Input: part model. Units: mm. Frame: model coordinates. Give positions to 0.01 mm unless a question says otherwise; leave off trailing zeros. Loops run counter-clockwise (first coordinate to the right, second up) from the corner with the lowest first, then second, coordinate; pieces in that order, holes last. Notation, with made-up numbers: (33.5, 55.25) - (87.5, 55.25) arc R36 cw to (87.5, 93.25) - close; hole circle Ø5 at (-7.5, 62). An arc over 180 degrees is marked (long way). Answer as a JSON object with one key per item and string values. Group by question number.
(1) Pin query (flat end, axial travel): P1, Ø1.8, axis at x = -85, y = 10, coming from the -Z side; P2, Ø2, axis at x = 22, z = 74.5, coming from the +Y side; P3, Ø2.5, axis at y = 13.5, z = 98, coming from the +X side; P4, Ø5, axis at y = 10.5, z = -56.5, coming from the +X side. Return the tip coordinate at first contact, or that it passes through.
(2) Section query B-B (z = 69.5). Return loops of the section in (x, y).
(3) Material intervals for L1, parallel to Y at x = -17.5, z = 97.9; L2, parallel to X at y = 2.3, z = -30; L3, parallel to Y at x = -96.15, z = -90, sorted ascending.
(4) Section query A-A (x = -65.5). Return loops of the section in (y, z).
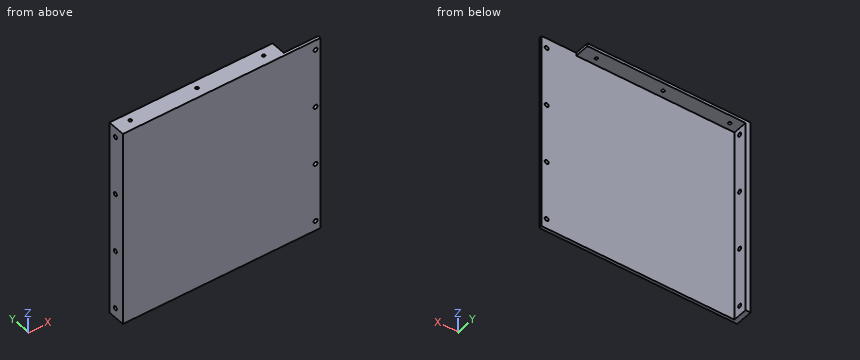
```python
from build123d import *

# Parameters (mm, degrees)
SKETCH1_W           = 200
SKETCH1_H           = 200
BOSS_EXTRUDE1_DEPTH = 3
SKETCH2_W           = 5
SKETCH2_H           = 200
BOSS_EXTRUDE2_DEPTH = 15
CUT_EXTRUDE1_REACH  = 226.33
SKETCH3_R           = 2
LPATTERN1_COUNT     = 4
LPATTERN1_PITCH     = 60
CUT_EXTRUDE2_REACH  = 144.215
SKETCH4_R           = 2
LPATTERN2_COUNT     = 4
LPATTERN2_PITCH     = 60
SKETCH5_W           = 160
SKETCH5_H           = 3
BOSS_EXTRUDE3_DEPTH = 15
CUT_EXTRUDE3_REACH  = 226.33
SKETCH6_R           = 1.5


with BuildPart() as part:
    # Sketch1 → Boss-Extrude1 (new body)
    with BuildSketch(Plane(origin=(0, 0, 0), x_dir=(1, 0, 0), z_dir=(0, 1, 0))):
        Rectangle(SKETCH1_W, SKETCH1_H)
    extrude(amount=BOSS_EXTRUDE1_DEPTH)

    # Sketch2 → Boss-Extrude2 (add)
    with BuildSketch(Plane(origin=(0, 3, 0), x_dir=(1, 0, 0), z_dir=(0, 1, 0))):
        with Locations((-97.5, 0)):
            Rectangle(SKETCH2_W, SKETCH2_H)
    extrude(amount=BOSS_EXTRUDE2_DEPTH)

    # Sketch3 → Cut-Extrude1 (cut, up to next)
    with BuildSketch(Plane.ZY.offset(100), mode=Mode.PRIVATE) as cut_extrude1_sk1:
        with Locations((90, 10)):
            Circle(SKETCH3_R)
    cut_extrude1_tool1 = extrude(cut_extrude1_sk1.sketch, amount=-CUT_EXTRUDE1_REACH, mode=Mode.PRIVATE) & part.part
    cut_extrude1 = cut_extrude1_tool1.solids().sort_by_distance((-100, 10, 90))[0]
    add(cut_extrude1, mode=Mode.SUBTRACT)

    # LPattern1: Cut-Extrude1 ×4
    with Locations(*[(0, 0, -i * LPATTERN1_PITCH) for i in range(1, LPATTERN1_COUNT)]):
        add(cut_extrude1, mode=Mode.SUBTRACT)

    # Sketch4 → Cut-Extrude2 (cut, up to next)
    with BuildSketch(Plane(origin=(0, 3, 0), x_dir=(1, 0, 0), z_dir=(0, 1, 0)), mode=Mode.PRIVATE) as cut_extrude2_sk1:
        with Locations(Location((95, 90, 0), (0, 0, 270))):
            Circle(SKETCH4_R)
    cut_extrude2_tool1 = extrude(cut_extrude2_sk1.sketch, amount=-CUT_EXTRUDE2_REACH, mode=Mode.PRIVATE) & part.part
    cut_extrude2 = cut_extrude2_tool1.solids().sort_by_distance((95, 3, -90))[0]
    add(cut_extrude2, mode=Mode.SUBTRACT)

    # LPattern2: Cut-Extrude2 ×4
    with Locations(*[(0, 0, i * LPATTERN2_PITCH) for i in range(1, LPATTERN2_COUNT)]):
        add(cut_extrude2, mode=Mode.SUBTRACT)

    # Sketch5 → Boss-Extrude3 (add)
    with BuildSketch(Plane(origin=(0, 3, 0), x_dir=(1, 0, 0), z_dir=(0, 1, 0))):
        with Locations((-15, -98.5)):
            Rectangle(SKETCH5_W, SKETCH5_H)
    extrude(amount=BOSS_EXTRUDE3_DEPTH)

    # Sketch6 → Cut-Extrude3 (cut, up to next)
    with BuildSketch(Plane.XY.offset(100), mode=Mode.PRIVATE) as cut_extrude3_sk1:
        with Locations((-85, 10)):
            Circle(SKETCH6_R)
    cut_extrude3_tool1 = extrude(cut_extrude3_sk1.sketch, amount=-CUT_EXTRUDE3_REACH, mode=Mode.PRIVATE) & part.part
    # Sketch6 → Cut-Extrude3 (cut, up to next)
    with BuildSketch(Plane.XY.offset(100), mode=Mode.PRIVATE) as cut_extrude3_sk2:
        with Locations((-17.5, 10)):
            Circle(SKETCH6_R)
    cut_extrude3_tool2 = extrude(cut_extrude3_sk2.sketch, amount=-CUT_EXTRUDE3_REACH, mode=Mode.PRIVATE) & part.part
    # Sketch6 → Cut-Extrude3 (cut, up to next)
    with BuildSketch(Plane.XY.offset(100), mode=Mode.PRIVATE) as cut_extrude3_sk3:
        with Locations((50, 10)):
            Circle(SKETCH6_R)
    cut_extrude3_tool3 = extrude(cut_extrude3_sk3.sketch, amount=-CUT_EXTRUDE3_REACH, mode=Mode.PRIVATE) & part.part
    add(cut_extrude3_tool1.solids().sort_by_distance((-85, 10, 100))[0], mode=Mode.SUBTRACT)
    add(cut_extrude3_tool2.solids().sort_by_distance((-17.5, 10, 100))[0], mode=Mode.SUBTRACT)
    add(cut_extrude3_tool3.solids().sort_by_distance((50, 10, 100))[0], mode=Mode.SUBTRACT)


solid = part.part
```
Recorded:
{
 "1": {"P1": "passes through", "P2": "stops at y = 3", "P3": "stops at x = 65", "P4": "stops at x = -95"},
 "2": {"outline": "(-100, 0) - (100, 0) - (100, 3) - (-95, 3) - (-95, 18) - (-100, 18) - close"},
 "3": {"L1": "y = 0 to 8.5, 11.5 to 18", "L2": "x = -100 to 93, 97 to 100", "L3": "y = 0 to 8, 12 to 18"},
 "4": {"outline": "(0, -100) - (3, -100) - (3, 97) - (18, 97) - (18, 100) - (0, 100) - close"}
}
